Work out the finished part from the listing and answer in its coordinate system (mm). Face numbers are marked on the shaded views. A direction names the side the tool comes from. Give positions to 0.01 mm unless a question says otherwise; leave off trailing zeros. Loops run counter-clockwise (first coordinate to the right, second up) from the corner with the lowest first, then second, coordinate; pieces in that order, holes last. Notation, with made-up numbers: (50, 66) - (60, 66) arc R25 ccw to (60, 90) - close; hole circle Ø3 at (33, -20.5). An arc over 180 degrees is marked (long way). One line per question, with ' | ' between items.
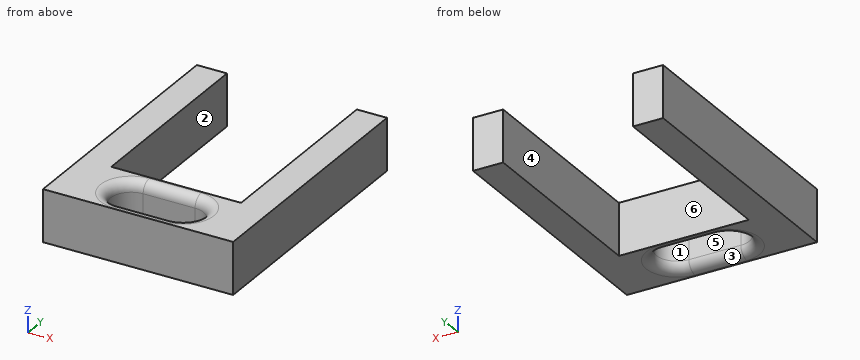
from build123d import *

# Parameters (mm, degrees)
BOSS_EXTRUDE1_DEPTH = 25.4
FILLET1_R           = 5


with BuildPart() as part:
    # Sketch1 → Boss-Extrude1 (new body)
    with BuildSketch(Plane.XY):
        Polygon((-46.5, 0), (-31.75, 0), (-31.75, -96.52), (31.75, -96.52), (31.75, 0), (46.5, 0), (46.5, -128.27), (-46.5, -128.27), align=None)
        with BuildLine():
            Line((-12.7, -102.395), (12.7, -102.395))
            ThreePointArc((12.7, -102.395), (22.7, -112.395), (12.7, -122.395))
            Line((12.7, -122.395), (-12.7, -122.395))
            ThreePointArc((-12.7, -122.395), (-22.7, -112.395), (-12.7, -102.395))
        make_face(mode=Mode.SUBTRACT)
    extrude(amount=BOSS_EXTRUDE1_DEPTH)

    # Fillet1
    fillet1_edges = [part.edges().sort_by_distance(p)[0] for p in [
        (-22.7, -112.395, 0),
        (0, -122.395, 0),
        (22.7, -112.395, 0),
        (0, -102.395, 0),
        (-22.7, -112.395, 25.4),
        (0, -122.395, 25.4),
        (22.7, -112.395, 25.4),
        (0, -102.395, 25.4),
    ]]
    fillet(fillet1_edges, radius=FILLET1_R)


solid = part.part
1. Find section B-B on x = -6. Write down the section's boundary in (y, z) (3 decimals), then the cut area to 3 significant figures.
Evaluation:
outline: (-128.27, 0) - (-127.395, 0) arc R5 ccw to (-122.395, 5) - (-122.395, 20.4) arc R5 ccw to (-127.395, 25.4) - (-128.27, 25.4) - close; (-102.395, 5) arc R5 ccw to (-97.395, 0) - (-96.52, 0) - (-96.52, 25.4) - (-97.395, 25.4) arc R5 ccw to (-102.395, 20.4) - close | area: 277 mm2
2. Determine the mould class of the marked faces 4, 5 and 6 for opening direction Y: +Y half, -Y half, draft (parallel to the pull), parting line (faces both ways), or undercut.
Evaluation:
face 4: draft | face 5: undercut | face 6: +Y half
3. Which of the six approach directions +Z, -Z, +X, -X, +Y, -Y give full straight-line access (tool end or side, diameter ignored) to the marked faces 1, 2 and 3?
Evaluation:
face 1: +Z, -Z | face 2: +Z, -Z, +Y | face 3: -Z
4. Find section C-C on z = 8.25. Write down the section's boundary in (x, y) (3 decimals), then the cut area to 3 significant figures.
Evaluation:
outline: (-46.5, -128.27) - (46.5, -128.27) - (46.5, 0) - (31.75, 0) - (31.75, -96.52) - (-31.75, -96.52) - (-31.75, 0) - (-46.5, 0) - close; hole (-12.7, -122.395) - (12.7, -122.395) arc R10 ccw to (12.7, -102.395) - (-12.7, -102.395) arc R10 ccw to start | area: 4,980 mm2
5. Find section A-A on y = -78.5. Write down the section's boundary in (x, z).
Evaluation:
outline: (-46.5, 0) - (-31.75, 0) - (-31.75, 25.4) - (-46.5, 25.4) - close; (31.75, 0) - (46.5, 0) - (46.5, 25.4) - (31.75, 25.4) - close
6. Consider L1, parallel to X at y = -46, z = 22; L2, parallel to Y at x = 8, z = 11.25 (3 decimals); L3, parallel to X at y = -113.5, z = 22.5. Determine where each line is inside the solid, lowest interval first.
Evaluation:
L1: -46.5 to -31.75, 31.75 to 46.5 | L2: -128.27 to -122.395, -102.395 to -96.52 | L3: -46.5 to -23.1, 23.1 to 46.5
7. A flat-ended cylindrical pin translates along its axis: pin 1 (5 mm diameter, centred on x = 3, z = 18.5, fed in from +Y). Find the tip coordinate at first contact, or state that the pin passes through.
Evaluation:
pin 1: y = -96.52
